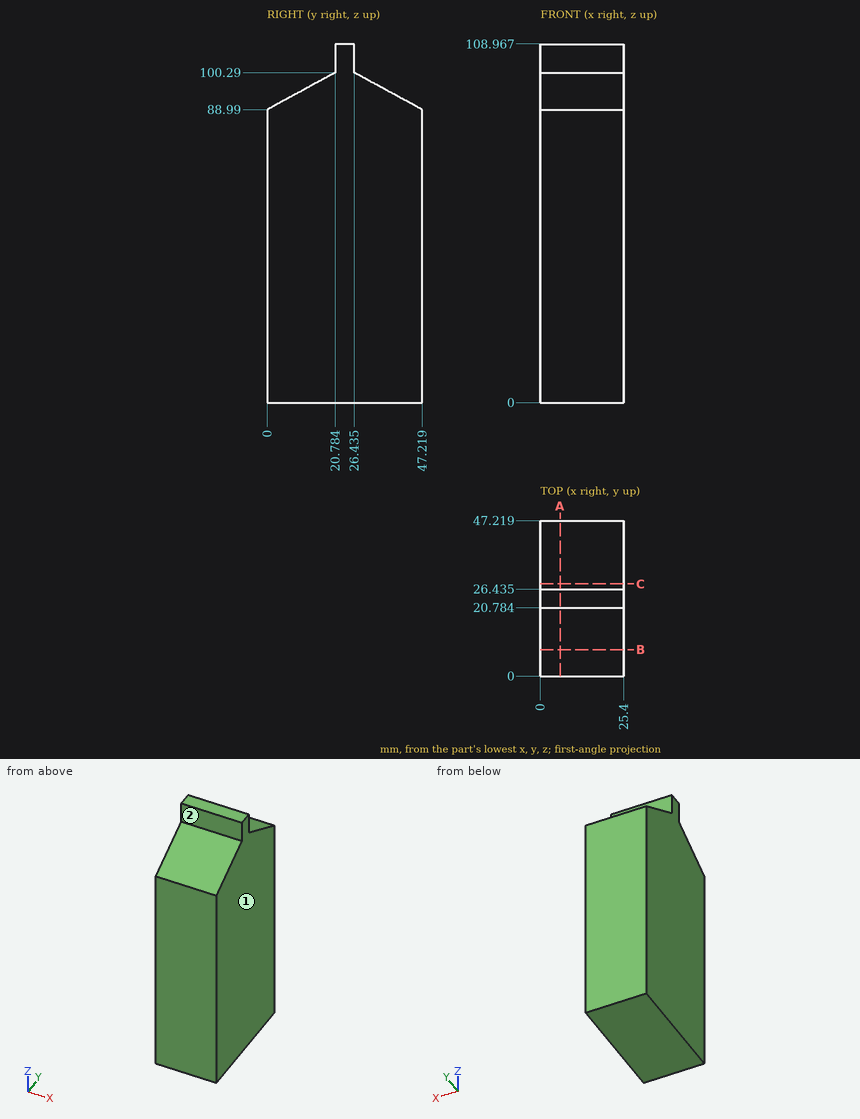
Here's the drawing with two shaded views (mm, measured from the low corner). I have some questions. A direction names the side the tool comes from. Coordinates: 2 decimals unless noted, no trailing zeros. Write each loop counter-clockwise with the first axis right and the second up, starting at its lowest first coordinate (ties: lowest second). Pieces come first, ordered by that corner, then holes. Notation, with made-up numbers: (79, 9) -> (93, 9) arc R27 ccw to (93, 27) -> close; hole circle Ø8 at (48.25, -14.5). An arc over 180 degrees is marked (long way). Use a Markdown table: item, result. Add a question column.
(1) If we section it at A-A, the plane x = 6: Write out the boundary of the cut face in (y, z) (1 decimal).
(2) Please list where these lines run through material, in increasing order: line 1 (Y direction, x = 24, z = 103) (1 decimal); line 2 (Y direction, x = 3.5, z = 93) (1 decimal); line 3 (Z direction, x = 19, y = 8.5).
(3) If we section it at B-B, the plane y = 8: Write out the boundary of the cut face in (x, z), and give its area (3 significant figures).
(4) I'm going to push flat-ended pins straight in: P1, Ø8, axis at x = 5, y = 42.5, coming from the +Z side; P2, Ø9.5, axis at x = 12.5, z = 106, coming from the -Y side; P3, Ø2.5, axis at x = 11, z = 105.5, coming from the +Y side (1 decimal). Where does each tip first touch, or does it pass through?
(5) For the marked faces 1 and 2, which set-ups out of +Z, -Z, +X, -X, +Y, -Y let a thin tool reach every point of the face, with its end or its side?
(6) If we section it at C-C, the plane y = 28: Write out the boundary of the cut face in (x, z), and give its area (3 significant figures).
Outcome:
| question | item | result |
|---|---|---|
| 1 | outline | (0, 0) -> (47.2, 0) -> (47.2, 89) -> (26.4, 100.3) -> (26.4, 109) -> (20.8, 109) -> (20.8, 100.3) -> (0, 89) -> close |
| 2 | line 1 | y = 20.8 to 26.4 |
| 2 | line 2 | y = 7.4 to 39.8 |
| 2 | line 3 | z = 0 to 93.61 |
| 3 | outline | (0, 0) -> (25.4, 0) -> (25.4, 93.34) -> (0, 93.34) -> close |
| 3 | area | 2,370 mm^2 |
| 4 | P1 | stops at z = 93.73 |
| 4 | P2 | stops at y = 20.78 |
| 4 | P3 | stops at y = 26.4 |
| 5 | face 1 | +Z, -Z, +X, +Y, -Y |
| 5 | face 2 | +Z, +X, -X, -Y |
| 6 | outline | (0, 0) -> (25.4, 0) -> (25.4, 99.44) -> (0, 99.44) -> close |
| 6 | area | 2,530 mm^2 |
